Input: dimensioned drawing with shaded views. Units: mm. Origin: part minimum x, y, z. Coordinates: 2 decimals unless noted, no trailing zeros. Loops run counter-clockwise (first coordinate to the right, second up) from the corner with the lowest first, then second, coordinate; pieces in that order, holes last. Notation, with made-up numbers: (-25.75, 27.5) - (0.25, 27.5) arc R33 cw to (0.25, 55.5) - close; hole circle Ø11 at (-38.75, 62). An arc over 180 degrees is marked (long way). Use one line per item in the form item = value. Start each with the question number.
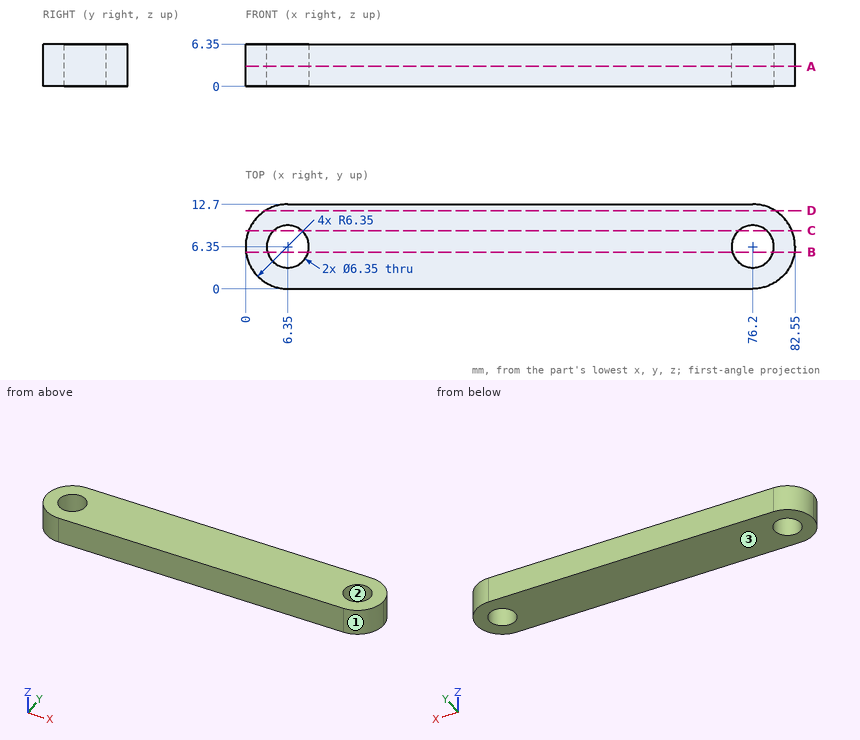
(1) Cut plane A-A, the plane z = 3. State how many separate pieces and enclosed holes the cut face has, plus the area to 3 significant figures.
(2) Contact query for a flat-ended pin moving along its axis: pin 1 (5.5 mm diameter, centred on x = 6.35, y = 6.35, fed in from -Z). Output: stop coordinate, or through.
(3) Cut plane D-D, the plane y = 11.75. Output: boundary loops of the cut face in (x, z), plus the area to 3 significant figures.
(4) Cut plane C-C, the plane y = 8.75. Output: boundary loops of the cut face in (x, z).
(5) Mould query, pull axis X, two halves, no side actions, for the marked faces 1, 2 and 3. Classes: +X half, -X half, draft (parallel to the pull), parting line (faces both ways), or undercut.
(6) Cut plane B-B, the plane y = 5.5. Output: boundary loops of the cut face in (x, z), plus the area to 3 significant figures.
(7) Material intervals for line 1 (Y direction, x = 6.35, z = 3.75) (3 decimals); line 2 (X direction, y = 8.25, z = 2.5); line 3 (X direction, y = 4, z = 3) (1 decimal), sorted ascending.
Recorded:
q1.separate_pieces = 1
q1.enclosed_holes = 2
q1.area = 950 mm²
q2.pin_1 = through
q3.outline = (3.01, 0) - (79.54, 0) - (79.54, 6.35) - (3.01, 6.35) - close
q3.area = 486 mm²
q4.outline = (0.47, 0) - (4.27, 0) - (4.27, 6.35) - (0.47, 6.35) - close; (8.43, 0) - (74.12, 0) - (74.12, 6.35) - (8.43, 6.35) - close; (78.28, 0) - (82.08, 0) - (82.08, 6.35) - (78.28, 6.35) - close
q5.face_1 = +X half
q5.face_2 = undercut
q5.face_3 = draft
q6.outline = (0.06, 0) - (3.29, 0) - (3.29, 6.35) - (0.06, 6.35) - close; (9.41, 0) - (73.14, 0) - (73.14, 6.35) - (9.41, 6.35) - close; (79.26, 0) - (82.49, 0) - (82.49, 6.35) - (79.26, 6.35) - close
q6.area = 446 mm²
q7.line_1 = 0 to 3.175, 9.525 to 12.7
q7.line_2 = 0.29 to 3.81, 8.89 to 73.66, 78.74 to 82.26
q7.line_3 = 0.5 to 4.2, 8.5 to 74.1, 78.3 to 82.1
